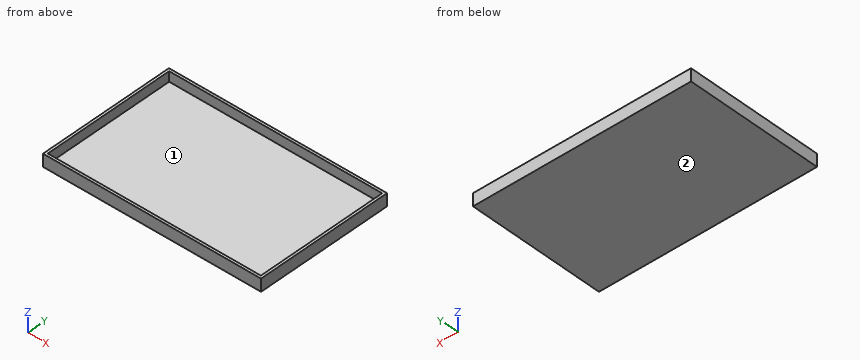
from build123d import *

# Parameters (mm, degrees)
F0_W     = 222.25
F0_H     = 139.7
F1_DEPTH = 12.7
F2_DEPTH = 12.7
F3_T     = -2.54


with BuildPart() as f1:
    # F0 (on Top) → F1 (new body)
    with BuildSketch(Plane.XY):
        with Locations((1.78089, -31.92896)):
            Rectangle(F0_W, F0_H)
    extrude(amount=F1_DEPTH)

    # F0 (on Top) → F2 (join)
    with BuildSketch(Plane.XY):
        with Locations((1.78089, -31.92896)):
            Rectangle(F0_W, F0_H)
    extrude(amount=F2_DEPTH)

    # F3
    f3_openings = [f1.faces().sort_by_distance(p)[0] for p in [
        (1.78089, -31.92896, 12.7),
    ]]
    offset(amount=F3_T, openings=f3_openings)


solid = f1.part
Work out the finished part from the listing and answer in its coordinate system (mm). Face numbers are marked on the shaded views. Give positions to 0.01 mm unless a question says otherwise; leave off trailing zeros. Order: outer loops, then holes, each group sorted by start corner. A loop starts at its lowest first (then second) coordinate and runs counter-clockwise, first axis right, second up. Notation, with made-up numbers: (46.25, 24.25) -> (105.25, 24.25) arc R23 ccw to (105.25, 34.25) -> close; hole circle Ø4 at (-6, 2). An arc over 180 degrees is marked (long way). Answer as a JSON object with one key per item and string values. Group by question number.
1. Consider line 1 along Y through (x, z) = (27, 9.25); line 2 along X through (y, z) = (-89, 5.25); line 3 along Z through (x, y) = (-70, -29.5). Determine where each line is inside the solid, lowest interval first. Write a range as [from, to].
2. The mould has two halves that part along X. Classify the marked faces 1 and 2: released by +X, released by -X, zero draft, split by the parting line, or undercut.
3. A flat-ended cylindrical pin translates along its axis: pin 1 Ø1 at (x, y) = (77.5, -56.5) entering from +Z. Find the tip coordinate at first contact, or state that the pin passes through.
4. Section C-C on y = -2 is taken. Determine the outline of the cut face in (x, z).
5. Section B-B on x = -48 is taken. Determine the outline of the cut face in (y, z).
6. Section A-A on z = 7.75 is taken. Determine the outline of the cut face in (x, y).
Result sheet:
{
 "1": {"line 1": "y = [-101.78, -99.24], [35.38, 37.92]", "line 2": "x = [-109.34, -106.8], [110.37, 112.91]", "line 3": "z = [0, 2.54]"},
 "2": {"face 1": "undercut", "face 2": "zero draft"},
 "3": {"pin 1": "stops at z = 2.54"},
 "4": {"outline": "(-109.34, 0) -> (112.91, 0) -> (112.91, 12.7) -> (110.37, 12.7) -> (110.37, 2.54) -> (-106.8, 2.54) -> (-106.8, 12.7) -> (-109.34, 12.7) -> close"},
 "5": {"outline": "(-101.78, 0) -> (37.92, 0) -> (37.92, 12.7) -> (35.38, 12.7) -> (35.38, 2.54) -> (-99.24, 2.54) -> (-99.24, 12.7) -> (-101.78, 12.7) -> close"},
 "6": {"outline": "(-109.34, -101.78) -> (112.91, -101.78) -> (112.91, 37.92) -> (-109.34, 37.92) -> close; hole (-106.8, -99.24) -> (110.37, -99.24) -> (110.37, 35.38) -> (-106.8, 35.38) -> close"}
}
